```python
from build123d import *

# Parameters (mm, degrees)
CUT_EXTRUDE1_DEPTH = 10
CIRPATTERN1_COUNT  = 3


with BuildPart() as part:
    # Sketch1 → Head Revolve (revolve)
    with BuildSketch(Plane.XY, mode=Mode.PRIVATE) as head_revolve_sk:
        with BuildLine():
            Line((0, 8.861467442), (0, 9.761467442))
            Line((0, 9.761467442), (1.6, 9.761467442))
            Line((1.6, 9.761467442), (1.6, 11.761467442))
            Line((1.6, 11.761467442), (2.796868049, 11.761467442))
            Line((2.796868049, 11.761467442), (2.796868049, 9.961467442))
            Line((2.796868049, 9.961467442), (2.809886353, 9.966286057))
            ThreePointArc((2.809886353, 9.966286057), (4.371289555, 9.767199261), (5.1, 8.371994401))
            Line((5.1, 8.371994401), (5.1, 3.155002023))
            ThreePointArc((5.1, 3.155002023), (4.556524041, 1.909027648), (3.273585714, 1.459708707))
            Line((3.273585714, 1.459708707), (3.25, 1.461467442))
            Line((3.25, 1.461467442), (3.25, 0.361467442))
            Line((3.25, 0.361467442), (2.45, 0.361467442))
            Line((2.45, 0.361467442), (2.45, 8.861467442))
            Line((2.45, 8.861467442), (0, 8.861467442))
        make_face()
    revolve(head_revolve_sk.sketch.rotate(Axis((0, 0, 0), (0, 1, 0)), 90), axis=Axis((0, 0, 0), (0, 1, 0)))

    # Sketch2 → Cut-Extrude1 (cut)
    with BuildSketch(Plane(origin=(0, 9.761467442, 0), x_dir=(1, 0, 0), z_dir=(0, 1, 0))):
        with BuildLine():
            Line((-0.42, 1.543891188), (-0.42, 0.242487113))
            Line((-0.42, 0.242487113), (-1.547048989, -0.408214924))
            ThreePointArc((-1.547048989, -0.408214924), (-1.385640646, 0.8), (-0.42, 1.543891188))
        make_face()
    cut_extrude1 = extrude(amount=-CUT_EXTRUDE1_DEPTH, mode=Mode.SUBTRACT)

    # CirPattern1: Cut-Extrude1 ×3 about axis
    cirpattern1_axis = Axis((0, 0, 0), (0, 1, 0))
    for i in range(1, CIRPATTERN1_COUNT):
        add(cut_extrude1.rotate(cirpattern1_axis, i * 360 / CIRPATTERN1_COUNT), mode=Mode.SUBTRACT)


solid = part.part
```
CAD build for the part. Positions are in the model's coordinates, mm. A direction names the side the tool comes from. Coordinates: 2 decimals unless noted, no trailing zeros. Order: outer loops, then holes, each group sorted by start corner. A loop starts at its lowest first (then second) coordinate and runs counter-clockwise, first axis right, second up. Notation, with made-up numbers: (30.25, 68.25) -> (43.25, 68.25) arc R8 cw to (43.25, 78.25) -> close; hole circle Ø11 at (31.25, 84.25). An arc over 180 degrees is marked (long way). Use one line per item in the form item = value. Start each with the question number.
1) Band-saw the part on A-A on z = 0. Give the cut face in (x, y) (3 decimals).
2) Drill centre lines: L1, parallel to X at y = 4.75, z = 0; L2, parallel to X at y = 10.9, z = 0; L3, parallel to Y at x = 1.25, z = -1.5. Where is each one in solid material? Low to high. Write a range as [from, to].
3) Drop flat-ended pins along their axis: pin 1 (1 mm diameter, centred on x = -0.5, z = 0, fed in from +Y); pin 2 (1 mm diameter, centred on y = 9, z = -1, fed in from -X); pin 3 (0.7 mm diameter, centred on y = 9.5, z = -1, fed in from +X). Give the stop position or say it passes through.
4) Tool access for faces 1 (the flat face through (0, 8.861, 0)), 2 (the flat face through (0.42, 9.3, -0.9)), 3 (the cylindrical face through (2.73, 10.85, 0.61)): list every direction of +Z, -Z, +X, -X, +Y, -Y with a clear straight run to the whole face (end or side of a thin tool).
5) Band-saw the part on B-B on y = 4.75. Give the cut face in (x, z), then the cut area to 3 significant figures.
6) Pull direction Z, two halves, no side cores. Call faces 4 (the flat face through (0, 9.761, 0)), 5 (the flat face through (2, 11.761, 0)), 6 (the cylindrical face through (1.978, 0.904, 2.579)): +Z half, -Z half, draft (parallel to the pull), parting line (faces both ways), or undercut.
Entries:
q1.outline = (-5.1, 3.155) arc R1.7 ccw to (-3.274, 1.46) -> (-3.25, 1.461) -> (-3.25, 0.361) -> (-2.45, 0.361) -> (-2.45, 8.861) -> (-1.6, 8.861) -> (-1.6, 11.761) -> (-2.797, 11.761) -> (-2.797, 9.961) -> (-2.81, 9.966) arc R1.7 ccw to (-5.1, 8.372) -> close; (-0.84, 8.861) -> (0.84, 8.861) -> (0.84, 9.761) -> (-0.84, 9.761) -> close; (1.6, 8.861) -> (2.45, 8.861) -> (2.45, 0.361) -> (3.25, 0.361) -> (3.25, 1.461) -> (3.274, 1.46) arc R1.7 ccw to (5.1, 3.155) -> (5.1, 8.372) arc R1.7 ccw to (2.81, 9.966) -> (2.797, 9.961) -> (2.797, 11.761) -> (1.6, 11.761) -> close
q2.L1 = [-5.1, -2.45], [2.45, 5.1]
q2.L2 = [-2.8, -1.6], [1.6, 2.8]
q2.L3 = [8.86, 11.76]
q3.pin_1 = 9.76
q3.pin_2 = -5.04
q3.pin_3 = 4.82
q4.face_1 = -Y
q4.face_2 = +Y, -Y
q4.face_3 = +Y
q5.outline = circle Ø10.2 at (0, 0); hole circle Ø4.9 at (0, 0)
q5.area = 62.9 mm2
q6.face_4 = undercut
q6.face_5 = draft
q6.face_6 = parting line
